from build123d import *

# Parameters (mm, degrees)
SKETCH1_R             = 5
BOSS_EXTRUDE1_DEPTH   = 11
M3_TAPPED_HOLE1_D     = 2.5
M3_TAPPED_HOLE1_DEPTH = 7.5
M3_TAPPED_HOLE1_TIP   = 0.751075774
CHAMFER2_SIZE         = 0.5


with BuildPart() as part:
    # Sketch1 → Boss-Extrude1 (new body)
    with BuildSketch(Plane.XY):
        Circle(SKETCH1_R)
    extrude(amount=BOSS_EXTRUDE1_DEPTH)

    # M3 Tapped Hole1
    with Locations(Plane(origin=(0, 0, 0), x_dir=(-1, 0, 0), z_dir=(0, 0, -1))):
        with Locations((0, 0)):
            Hole(M3_TAPPED_HOLE1_D / 2, depth=M3_TAPPED_HOLE1_DEPTH)
            with Locations((0, 0, -(M3_TAPPED_HOLE1_DEPTH + M3_TAPPED_HOLE1_TIP / 2))):  # 118° drill point
                Cone(0, M3_TAPPED_HOLE1_D / 2, M3_TAPPED_HOLE1_TIP, mode=Mode.SUBTRACT)

    # Chamfer2
    chamfer2_edges = [part.edges().sort_by_distance(p)[0] for p in [
        (-5, 0, 0),
        (-5, 0, 11),
    ]]
    chamfer(chamfer2_edges, length=CHAMFER2_SIZE)


solid = part.part
Part model, mm, in its own coordinate system. Coordinates: 2 decimals unless noted, no trailing zeros. Loops run counter-clockwise (first coordinate to the right, second up) from the corner with the lowest first, then second, coordinate; pieces in that order, holes last. Notation, with made-up numbers: (6, 68) -> (56, 68) arc R22 cw to (56, 80) -> close; hole circle Ø9 at (-30.5, 81.5). An arc over 180 degrees is marked (long way). Use a Markdown table: item, result. Add a question column.
Item 1: Band-saw the part on A-A on z = 6.75. Write the cut outline in (x, y), plus the area to 3 significant figures.
Item 2: Band-saw the part on B-B on z = 8.5. Write the cut outline in (x, y), plus the area to 3 significant figures.
Item 3: Flat gauge pins, fed straight in: P1, Ø1.5, axis at x = 0, y = 0, coming from the -Z side; P2, Ø3, axis at x = 3, z = 8.5, coming from the +Y side; P3, Ø5, axis at x = 1, z = 6.5, coming from the -Y side; P4, Ø2, axis at y = -1.5, z = 1.5, coming from the -X side. Where does each tip first touch, or does it go through?
Item 4: Probe probe 1 along Y at (x, z) = (0, 4); probe 2 along X at (y, z) = (-0.5, 5.75); probe 3 along X at (y, z) = (0.75, 3.5). List the from-to ranges inside material, lowest first.
Item 5: Pull direction X, two halves, no side cores. Call faces 1 (the cylindrical face through (-1.08, -4.88, 5.43)), 2 (the cylindrical face through (-0.27, -1.22, 3.8)), 3 (the flat face through (0, 0, 11)): +X half, -X half, draft (parallel to the pull), parting line (faces both ways), or undercut.
Geometry says:
| question | item | result |
|---|---|---|
| 1 | outline | circle Ø10 at (0, 0); hole circle Ø2.5 at (0, 0) |
| 1 | area | 73.6 mm² |
| 2 | outline | circle Ø10 at (0, 0) |
| 2 | area | 78.5 mm² |
| 3 | P1 | z = 7.8 |
| 3 | P2 | y = 4.77 |
| 3 | P3 | y = -5 |
| 3 | P4 | x = -4.97 |
| 4 | probe 1 | -5 to -1.25, 1.25 to 5 |
| 4 | probe 2 | -4.97 to -1.15, 1.15 to 4.97 |
| 4 | probe 3 | -4.94 to -1, 1 to 4.94 |
| 5 | face 1 | parting line |
| 5 | face 2 | undercut |
| 5 | face 3 | draft |
